For this review, take the finished solid that the model builds, in its own axes (mm). A direction names the side the tool comes from. Give positions to 0.01 mm unless a question says otherwise; leave off trailing zeros. Order: outer loops, then holes, each group sorted by start corner. A loop starts at its lowest first (then second) coordinate and runs counter-clockwise, first axis right, second up. Notation, with made-up numbers: M 27,30.25 L 38,30.25 A15 cw 38,53.25 Z; hole C 20,75 d10. An arc over 180 degrees is marked long. Use CSV: the item, a comma, the result in double quotes. Start each with the question number.
(1) Consider section A-A (x = 23.5). Write out the cut boundary in (y, z).
(2) Consider section C-C (y = 3.75). Write out the cut boundary in (x, z).
(3) Wall thickness on L1, parallel to X at y = 1, z = 0.5; L2, parallel to X at y = 1, z = 1; L3, parallel to Z at x = 0, y = 4.5: over which ranges is each line inside the solid? List them lowest first. Write a range as from..to.
(4) Consider section D-D (x = 4). Write out the cut boundary in (y, z), and give its area (3 significant figures).
(5) Consider section B-B (z = 1.75). Write out the cut boundary in (x, y), and give its area (3 significant figures).
(6) Draft analysis for pull direction X (two halves, no side actions). For faces 1 (the face through (7.263, 3.549, 3.285)), 2 (the face through (22, 3.45, -0.26)), 3 (the face through (6, 7, 0)), 4 (the face through (18, 3.45, -0.26)), state which applies: pulls with the +X half, pulls with the -X half, needs draft (parallel to the pull), parting line crosses it, or undercut.
(7) Clearance check with flat-ended pins moving along their axes: P1, Ø1.5, axis at y = 2.5, z = 5.5, coming from the -X side; P2, Ø2.5, axis at x = 19.5, z = -0.2, coming from the -Y side; P3, Ø2, axis at x = 8, y = 2.5, coming from the +Z side. State where each tip first meets the part, or that it passes through.
(8) Tool access review of faces 5 (the face through (6, 0, 0)), 6 (the face through (17, 3, -2.96)): name each direction out of +Z, -Z, +X, -X, +Y, -Y from which nothing blocks a thin tool from reaching the whole face with its end or side.
```python
from build123d import *

# Parameters (mm, degrees)
SKETCH4_R           = 1.5
SKETCH4_R_2         = 3
BOSS_EXTRUDE1_DEPTH = 7
FILLET1_R           = 3


with BuildPart() as part:
    # Sketch4 → Boss-Extrude1 (new body)
    with BuildSketch(Plane(origin=(0, 0, 0), x_dir=(1, 0, 0), z_dir=(0, 1, 0))):
        with BuildLine():
            Line((6.89102232, 2.960373522), (24.66941446, 2.960373522))
            ThreePointArc((24.66941446, 2.960373522), (26.39916632, -0.573574214), (23.142085355, -2.780891971))
            Line((23.142085355, -2.780891971), (6.89102232, -2.960373522))
            ThreePointArc((6.89102232, -2.960373522), (4.125966468, -6.263098331), (0, -7.5))
            ThreePointArc((0, -7.5), (-7.5, 0), (0, 7.5))
            ThreePointArc((0, 7.5), (4.125966468, 6.263098331), (6.89102232, 2.960373522))
        make_face()
        with Locations((23.5, 0.197681027)):
            Circle(SKETCH4_R, mode=Mode.SUBTRACT)
        with Locations((19.5, 0.197681027)):
            Circle(SKETCH4_R, mode=Mode.SUBTRACT)
        Circle(SKETCH4_R_2, mode=Mode.SUBTRACT)
    extrude(amount=BOSS_EXTRUDE1_DEPTH)

    # Fillet1
    fillet1_edges = [part.edges().sort_by_distance(p)[0] for p in [
        (6.89102232, 3.5, -2.960373522),
        (6.89102232, 3.5, 2.960373522),
    ]]
    fillet(fillet1_edges, radius=FILLET1_R)


solid = part.part
```
Check result:
1,outline,"M 0,-2.96 L 7,-2.96 L 7,-1.7 L 0,-1.7 Z; M 0,1.3 L 7,1.3 L 7,2.8 L 0,2.8 Z"
2,outline,"M 6.17,-4.26 A3 cw 8.64,-2.96 L 24.67,-2.96 A3 ccw 23.14,2.78 L 8.62,2.94 A3 cw 6.18,4.24 A7.5 ccw long Z; hole C 0,0 d6; hole C 19.5,-0.2 d3; hole C 23.5,-0.2 d3"
3,L1,"x = -7.48..-2.96, 2.96..18.17, 20.83..22.17, 24.83..26.42"
3,L2,"x = -7.43..-2.83, 2.83..18.6, 20.4..22.6, 24.4..26.25"
3,L3,"z = -7.5..-3, 3..7.5"
4,outline,"M 0,-6.34 L 7,-6.34 L 7,6.34 L 0,6.34 Z"
4,area,"88.8 mm^2"
5,outline,"M -7.29,0 L -2.44,0 L -2.44,7 L -7.29,7 Z; M 2.44,0 L 25.78,0 L 25.78,7 L 2.44,7 Z"
5,area,"197 mm^2"
6,face 1,"pulls with the +X half"
6,face 2,"undercut"
6,face 3,"needs draft"
6,face 4,"undercut"
7,P1,"stops at x = -5.8"
7,P2,"passes through"
7,P3,"stops at z = 3.44"
8,face 5,"+Z, -Z, +X, -X, -Y"
8,face 6,"-Z, +X, +Y, -Y"
